The listing builds one solid part. Answer for the finished solid, in the listing's coordinates (mm). Give positions to 0.01 mm unless a question says otherwise; leave off trailing zeros. Order: outer loops, then holes, each group sorted by start corner. A loop starts at its lowest first (then second) coordinate and runs counter-clockwise, first axis right, second up. Notation, with made-up numbers: (86.25, 1.5) - (138.25, 1.5) arc R22 ccw to (138.25, 9.5) - close; hole circle Ø9 at (86.25, 81.5). An arc over 180 degrees is marked (long way). Answer in a Markdown table with one row per item.
Autodesk Inventor part; units mm, degrees
ref_plane "YZ Plane" through (0, 0, 0) normal (1, 0, 0) x (0, 1, 0)
ref_plane "XZ Plane" through (0, 0, 0) normal (0, 1, 0) x (-1, 0, 0)
ref_plane "XY Plane" through (0, 0, 0) normal (0, 0, 1) x (1, 0, 0)
sketch "Sketch1" plane through (0, 0, 0) normal (0, 1, 0) x (-1, 0, 0)
  line L0 (0, 0) -> (-614.3625, 0)
  line L1 (-614.3625, 0) -> (-614.3625, -228.6)
  line L2 (-614.3625, -228.6) -> (0, -228.6)
  line L3 (0, -228.6) -> (0, 0)
  dimension "d0" = 614.3625
  dimension "d1" = 228.6
extrude "Extrusion1" add sketch "Sketch1" along normal blind 6.35
sketch "Sketch2" plane through (0, 6.35, 0) normal (0, 1, 0) x (1, 0, 0)
  line L0 (0, 228.6) -> (0, 0)
  line L1 (0, 0) -> (307.1812, 0)
  line L2 (0, 0) -> (614.3625, 0)
  line L3 (307.1812, 0) -> (307.1812, 226.2221)
  line L4 (0, 0) -> (25.4, 0)
  line L5 (25.4, 0) -> (25.4, 25.4)
  line L6 (25.4, 25.4) -> (294.4812, 25.4)
  line L7 (294.4812, 25.4) -> (294.4812, 203.2)
  line L8 (294.4812, 203.2) -> (25.4, 203.2)
  line L9 (25.4, 203.2) -> (25.4, 25.4)
  line L10 (588.9625, 25.4) -> (319.8812, 25.4)
  line L11 (319.8812, 25.4) -> (319.8812, 203.2)
  line L12 (319.8812, 203.2) -> (588.9625, 203.2)
  line L13 (588.9625, 203.2) -> (588.9625, 25.4)
  dimension "d4" = 307.1812
  dimension "d5" = 25.4
  dimension "d6" = 25.4
  dimension "d7" = 269.0813
  dimension "d8" = 177.8
extrude "Extrusion2" cut sketch "Sketch2" against normal blind 117.475
sketch "Sketch3" plane through (0, 6.35, 0) normal (0, 1, 0) x (1, 0, 0)
  line L0 (614.3625, 228.6) -> (0, 228.6)
  line L1 (0, 228.6) -> (3.175, 228.6)
  line L2 (3.175, 228.6) -> (3.175, 0)
  line L3 (3.175, 0) -> (0, 0)
  line L4 (0, 0) -> (3.175, 0)
  line L5 (0, 228.6) -> (0, 0)
  line L6 (0, 228.6) -> (0, 0)
  dimension "d11" = 3.175
sketch "Sketch4" plane through (0, 6.35, 0) normal (0, 1, 0) x (1, 0, 0)
  line L0 (614.3625, 0) -> (614.3625, 228.6)
  line L1 (614.3625, 228.6) -> (611.1875, 228.6)
  line L2 (614.3625, 228.6) -> (0, 228.6)
  line L3 (611.1875, 228.6) -> (611.1875, 0)
  line L4 (611.1875, 0) -> (614.3625, 0)
  line L5 (614.3625, 0) -> (611.1875, 0)
  line L6 (614.3625, 228.6) -> (614.3625, 0)
  line L7 (294.4812, 25.4) -> (25.4, 25.4)
  line L8 (25.4, 203.2) -> (294.4812, 203.2)
  line L9 (294.4812, 203.2) -> (294.4812, 25.4)
  line L10 (25.4, 25.4) -> (25.4, 203.2)
  line L11 (25.4, 25.4) -> (25.4, 34.925)
  line L12 (25.4, 34.925) -> (294.4812, 34.925)
  line L13 (294.4812, 25.4) -> (294.4812, 34.925)
  line L14 (294.4812, 25.4) -> (25.4, 25.4)
  line L15 (25.4, 203.2) -> (294.4812, 203.2)
  line L16 (294.4812, 203.2) -> (294.4812, 193.675)
  line L17 (294.4812, 193.675) -> (25.4, 193.675)
  line L18 (25.4, 203.2) -> (25.4, 193.675)
  point P0 (0, 0)
  dimension "d12" = 3.175
  dimension "d20" = 177.8
  dimension "d21" = 269.0813
  dimension "d22" = 9.525
  dimension "d23" = 9.525
sketch "Sketch5" plane through (0, 6.35, 0) normal (0, 1, 0) x (1, 0, 0)
  line L0 (614.3625, 228.6) -> (0, 228.6)
  line L1 (0, 0) -> (614.3625, 0)
  line L2 (0, 228.6) -> (3.175, 228.6)
  line L3 (3.175, 228.6) -> (3.175, 0)
  line L4 (3.175, 0) -> (0, 0)
  line L5 (0, 0) -> (0, 228.6)
  line L6 (614.3625, 228.6) -> (611.1875, 228.6)
  line L7 (611.1875, 228.6) -> (611.1875, 0)
  line L8 (611.1875, 0) -> (614.3625, 0)
  line L9 (614.3625, 0) -> (614.3625, 228.6)
  dimension "d13" = 3.175
  dimension "d14" = 3.175
extrude "Extrusion3" cut sketch "Sketch5" against normal blind 25.4 contours L3 L1 L5 L0
sketch "Sketch6" plane through (0, 6.35, 0) normal (0, 1, 0) x (1, 0, 0)
  line L0 (3.175, 0) -> (614.3625, 0)
  line L1 (614.3625, 228.6) -> (611.1875, 228.6)
  line L2 (611.1875, 228.6) -> (611.1875, 0)
  line L3 (611.1875, 0) -> (614.3625, 0)
  line L4 (614.3625, 0) -> (614.3625, 228.6)
  point P0 (0, 0)
  dimension "d17" = 3.175
extrude "Extrusion4" cut sketch "Sketch6" against normal blind 25.4
extrude "Extrusion5" add sketch "Sketch4" against normal blind 6.35 contours L7 L10 L12 L9 | L17 L10 L8 L9
sketch "Sketch7" plane through (0, 6.35, 0) normal (0, 1, 0) x (1, 0, 0)
  line L0 (319.8812, 203.2) -> (319.8812, 25.4)
  line L1 (319.8812, 203.2) -> (319.8812, 193.675)
  line L2 (319.8812, 193.675) -> (588.9625, 193.675)
  line L3 (588.9625, 25.4) -> (588.9625, 203.2)
  line L4 (588.9625, 203.2) -> (588.9625, 193.675)
  line L5 (588.9625, 203.2) -> (319.8812, 203.2)
  line L6 (588.9625, 203.2) -> (319.8812, 203.2)
  line L7 (319.8812, 25.4) -> (588.9625, 25.4)
  line L8 (319.8812, 25.4) -> (319.8812, 34.925)
  line L9 (319.8812, 34.925) -> (588.9625, 34.925)
  line L10 (588.9625, 25.4) -> (588.9625, 34.925)
  line L11 (588.9625, 25.4) -> (319.8812, 25.4)
  point P0 (0, 0)
  dimension "d26" = 9.525
  dimension "d27" = 9.525
extrude "Extrusion6" add sketch "Sketch7" against normal blind 6.35 contours L5 L3 L2 L0 | L9 L3 L7 L0
sketch "Sketch8" plane through (0, 6.35, 0) normal (0, 1, 0) x (1, 0, 0)
  line L0 (611.1875, 0) -> (611.1875, 228.6)
  line L1 (3.175, 228.6) -> (3.175, 0)
  point P0 (0, 0)
  dimension "d30" = 608.0125
extrude "Extrusion7" add sketch "Sketch3" against normal blind 6.35
properties part number "BottomHalfofFront_Ocampo"
Item 1: Find section B-B on x = 97.5. Write down the section's boundary in (y, z) (3 decimals), then the cut area to 3 significant figures.
Answer block:
| item | result |
|---|---|
| outline | (0, -228.6) - (6.35, -228.6) - (6.35, -193.675) - (0, -193.675) - close; (0, -34.925) - (6.35, -34.925) - (6.35, 0) - (0, 0) - close |
| area | 444 mm² |
Item 2: Find section C-C on y = 2. Write down the section's boundary in (x, z) (1 decimal).
Answer block:
| item | result |
|---|---|
| outline | (0, -228.6) - (611.2, -228.6) - (611.2, 0) - (0, 0) - close; hole (25.4, -193.7) - (294.5, -193.7) - (294.5, -34.9) - (25.4, -34.9) - close; hole (319.9, -193.7) - (589, -193.7) - (589, -34.9) - (319.9, -34.9) - close |
Item 3: Consider line 1 (X direction, y = 4.75, z = -159.5); line 2 (Z direction, x = 447, y = 4) (3 decimals). Determine where each line is inside the solid, lowest interval first.
Answer block:
| item | result |
|---|---|
| line 1 | 0 to 25.4, 294.48 to 319.88, 588.96 to 611.19 |
| line 2 | -228.6 to -193.675, -34.925 to 0 |
Item 4: Find section A-A on z = -55. Write down the section's boundary in (x, y).
Answer block:
| item | result |
|---|---|
| outline | (0, 0) - (25.4, 0) - (25.4, 6.35) - (0, 6.35) - close; (294.48, 0) - (319.88, 0) - (319.88, 6.35) - (294.48, 6.35) - close; (588.96, 0) - (611.19, 0) - (611.19, 6.35) - (588.96, 6.35) - close |
